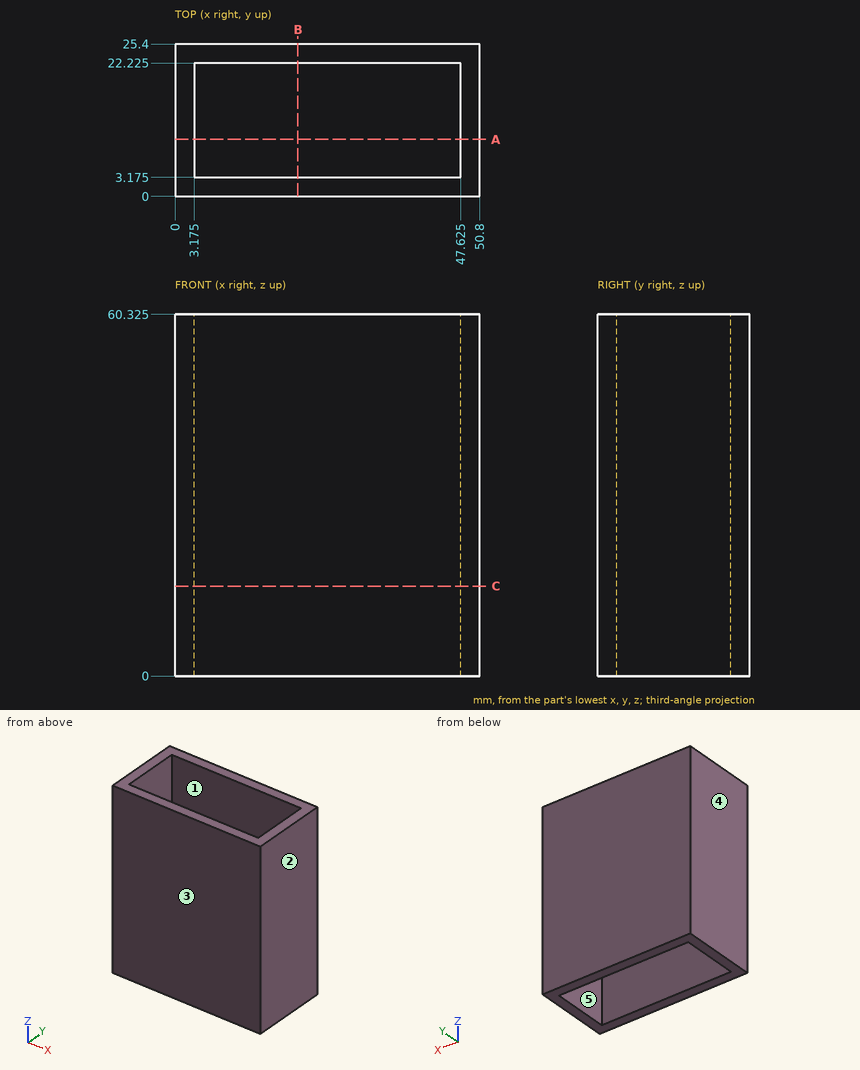
Answer from the drawing. Dimensions are ordinates in mm from the lowest x, y and z of the part. A direction names the side the tool comes from. Give positions to 0.01 mm unless a question says otherwise; leave off trailing zeros. Order: outer loops, then holes, each group sorted by start corner. A loop starts at its lowest first (then second) coordinate and runs counter-clockwise, first axis right, second up. Notation, with made-up numbers: (58, -29.75) - (117, -29.75) arc R16 ccw to (117, -11.75) - close; hole circle Ø6 at (62.5, 10). An arc over 180 degrees is marked (long way). One line per item, written item: value. Start each with the question number.
1) A cutting plane is placed at C-C on z = 15. Give the vertices of the cut face in (x, y) (3 decimals), then the cut area to 3 significant figures.
2) A cutting plane is placed at B-B on x = 20.5. Give the vertices of the cut face in (y, z) (3 decimals), then the cut area to 3 significant figures.
3) Find the intervals of material crossed by L1, parallel to X at y = 4.25, z = 55 (3 decimals); L2, parallel to Y at x = 27, z = 48 (3 decimals), in increasing order.
4) A tool of negligible diameter and unlimited length cuts with its end or side. For the marked faces 4 and 5, from which of +Z, -Z, +X, -X, +Y, -Y can it reach the whole face along a straight path? Write none if from no direction.
5) A cutting plane is placed at A-A on y = 9.5. Give the vertices of the cut face in (x, z) (3 decimals), then the cut area to 3 significant figures.
6) Given pin 1 Ø2 at (x, z) = (43.5, 50) entering from -Y, flat-ended and moving along its own axis, determine where the tip first touches the part or whether it passes through.
7) The mould has two halves that part along Y. Classify the marked faces 1, 2 and 3: released by +Y, released by -Y, zero draft, split by the parting line, or undercut.
Answer sheet:
1. outline: (0, 0) - (50.8, 0) - (50.8, 25.4) - (0, 25.4) - close; hole (3.175, 3.175) - (47.625, 3.175) - (47.625, 22.225) - (3.175, 22.225) - close
1. area: 444 mm2
2. outline: (0, 0) - (3.175, 0) - (3.175, 60.325) - (0, 60.325) - close; (22.225, 0) - (25.4, 0) - (25.4, 60.325) - (22.225, 60.325) - close
2. area: 383 mm2
3. L1: x = 0 to 3.175, 47.625 to 50.8
3. L2: y = 0 to 3.175, 22.225 to 25.4
4. face 4: +Z, -Z, -X, +Y, -Y
4. face 5: +Z, -Z
5. outline: (0, 0) - (3.175, 0) - (3.175, 60.325) - (0, 60.325) - close; (47.625, 0) - (50.8, 0) - (50.8, 60.325) - (47.625, 60.325) - close
5. area: 383 mm2
6. pin 1: stops at y = 0
7. face 1: undercut
7. face 2: zero draft
7. face 3: released by -Y
